Input: dimensioned drawing with shaded views. Units: mm. Origin: part minimum x, y, z. A direction names the side the tool comes from. Coordinates: 2 decimals unless noted, no trailing zeros. Order: outer loops, then holes, each group sorted by start corner. A loop starts at its lowest first (then second) coordinate and runs counter-clockwise, first axis right, second up. Notation, with made-up numbers: (27.25, 65) -> (39.25, 65) arc R21 ccw to (39.25, 88) -> close; hole circle Ø6 at (30.25, 4). An arc over 180 degrees is marked (long way). Write item = value, one per line. Start each with the question number.
Item 1: Set-up query: the marked faces 1, 2, 3 and 4. Return all of +Z, -Z, +X, -X, +Y, -Y with unobstructed straight access to the full face (end or side cutting, diameter ignored); none if empty.
Item 2: Section query C-C (z = 20.5). Output: boundary loops of the cut face in (x, y) (1 decimal), then the cut area to 3 significant figures.
Item 3: Section query B-B (x = 26.5). Output: boundary loops of the cut face in (y, z) (1 decimal).
Item 4: Section query D-D (x = 58). Output: boundary loops of the cut face in (y, z) (1 decimal).
Item 5: Contact query for flat-ended pins moving along their axis: pin 1 (5 mm diameter, centred on y = 62.5, z = 21.5, fed in from +X); pin 2 (4 mm diameter, centred on x = 43.5, z = 11.5, fed in from +Y); pin 3 (8 mm diameter, centred on y = 91, z = 12.5, fed in from -X) (1 decimal). Output: stop coordinate, or through.
Item 6: Mould query, pull axis X, two halves, no side actions, for the marked faces 5, 6 and 7. Classes: released by +X, released by -X, zero draft, split by the parting line, or undercut.
Item 7: Ray query, line 1 along X through (y, z) = (18.5, 11) (1 decimal); line 2 along X through (y, z) = (17.5, 19) (1 decimal); line 3 along X through (y, z) = (100, 14.5) (1 decimal). Return the intervals inside material, ascending. Write a range as [from, to].
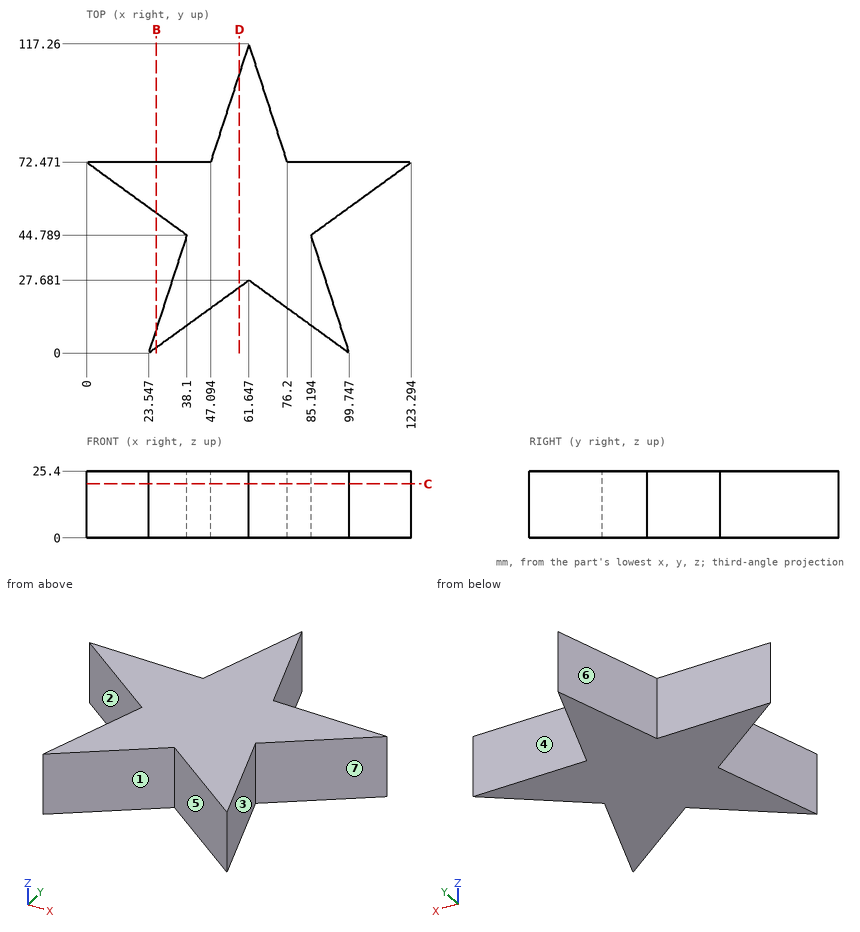
Computed:
q1.face_1 = +Z, -Z, -Y
q1.face_2 = +Z, -Z, -X
q1.face_3 = +Z, -Z, +X
q1.face_4 = +Z, -Z, +X, +Y
q2.outline = (0, 72.5) -> (38.1, 44.8) -> (23.5, 0) -> (61.6, 27.7) -> (99.7, 0) -> (85.2, 44.8) -> (123.3, 72.5) -> (76.2, 72.5) -> (61.6, 117.3) -> (47.1, 72.5) -> close
q2.area = 4,720 mm^2
q3.outline = (2.1, 0) -> (9.1, 0) -> (9.1, 25.4) -> (2.1, 25.4) -> close; (53.2, 0) -> (72.5, 0) -> (72.5, 25.4) -> (53.2, 25.4) -> close
q4.outline = (25, 0) -> (106, 0) -> (106, 25.4) -> (25, 25.4) -> close
q5.pin_1 = 113.01
q5.pin_2 = 72.47
q5.pin_3 = 51.8
q6.face_5 = undercut
q6.face_6 = released by -X
q6.face_7 = released by +X
q7.line_1 = [29.6, 49], [74.3, 93.7]
q7.line_2 = [29.2, 47.6], [75.7, 94.1]
q7.line_3 = [56, 67.3]
